```python
from build123d import *

# Parameters (mm, degrees)
SKETCH1_W           = 126
SKETCH1_H           = 126
BOSS_EXTRUDE1_DEPTH = 5
SKETCH3_R           = 12.5
BOSS_EXTRUDE2_DEPTH = 7.5
SKETCH4_R           = 2.95
CUT_EXTRUDE1_DEPTH  = 11.5
SKETCH6_R           = 2.5
CUT_EXTRUDE2_DEPTH  = 179.628805068
CHAMFER1_SIZE       = 10
CHAMFER1_SIZE_2     = 7.26542528
SKETCH8_W           = 13
SKETCH8_H           = 63.879672954
SKETCH8_H_2         = 19
CUT_EXTRUDE3_DEPTH  = 179.348675353
SKETCH9_R           = 30
CUT_EXTRUDE4_DEPTH  = 179.348675353
SKETCH11_W          = 2
SKETCH11_H          = 2
CUT_EXTRUDE5_DEPTH  = 3


with BuildPart() as part:
    # Sketch1 → Boss-Extrude1 (new body)
    with BuildSketch(Plane(origin=(0, 0, 0), x_dir=(1, 0, 0), z_dir=(0, 1, 0))):
        with Locations((63, 63)):
            Rectangle(SKETCH1_W, SKETCH1_H)
    extrude(amount=BOSS_EXTRUDE1_DEPTH)

    # Sketch3 → Boss-Extrude2 (add)
    with BuildSketch(Plane(origin=(0, 5, 0), x_dir=(1, 0, 0), z_dir=(0, 1, 0))):
        with Locations(Location((108.6, 108.6, 0), (0, 0, 90))):
            Circle(SKETCH3_R)
    extrude(amount=BOSS_EXTRUDE2_DEPTH)

    # Sketch4 → Cut-Extrude1 (cut)
    with BuildSketch(Plane.XZ):
        with Locations(Location((108.6, -108.6, 0), (0, 0, 270))):
            Circle(SKETCH4_R)
    extrude(amount=-CUT_EXTRUDE1_DEPTH, mode=Mode.SUBTRACT)

    # Sketch6 → Cut-Extrude2 (cut, through all)
    with BuildSketch(Plane(origin=(0, 12.5, 0), x_dir=(1, 0, 0), z_dir=(0, 1, 0))):
        with Locations(Location((108.6, 108.6, 0), (0, 0, 270))):
            Circle(SKETCH6_R)
    extrude(amount=-CUT_EXTRUDE2_DEPTH, mode=Mode.SUBTRACT)

    # Chamfer1
    # the kernel refuses this chamfer: 10, 7.26542528 mm, written as the material it takes off along each edge
    with BuildSketch(Plane(origin=(108.6, 12.5, -108.6), x_dir=(0, 0, -1), z_dir=(1, 0, 0))) as chamfer1_piece_1_section:
        Polygon((12.5, -CHAMFER1_SIZE), (12.5 - CHAMFER1_SIZE_2, 0), (12.5, 0), align=None)
    chamfer1_piece_1 = revolve(axis=Axis((108.6, 12.5, -108.6), (0, 1, 0)), mode=Mode.PRIVATE)
    chamfer1_piece_1 = split(chamfer1_piece_1, bisect_by=Plane(origin=(108.6, 5, -100.650989912), z_dir=(0, 1, 0)), keep=Keep.TOP, mode=Mode.PRIVATE)
    add(chamfer1_piece_1, mode=Mode.SUBTRACT)

    # Sketch8 → Cut-Extrude3 (cut, through all)
    with BuildSketch(Plane(origin=(0, 5, 0), x_dir=(1, 0, 0), z_dir=(0, 1, 0))):
        with Locations((107.763328316, 61.0093315)):
            Rectangle(SKETCH8_W, SKETCH8_H)
        with Locations((107.763328316, 14.5)):
            Rectangle(SKETCH8_W, SKETCH8_H_2)
    extrude(amount=-CUT_EXTRUDE3_DEPTH, mode=Mode.SUBTRACT)

    # Sketch9 → Cut-Extrude4 (cut, through all)
    with BuildSketch(Plane(origin=(0, 5, 0), x_dir=(1, 0, 0), z_dir=(0, 1, 0))):
        with Locations(Location((50.837155032, 48.974583989, 0), (0, 0, 270))):
            Circle(SKETCH9_R)
    extrude(amount=-CUT_EXTRUDE4_DEPTH, mode=Mode.SUBTRACT)

    # Sketch11 → Cut-Extrude5 (cut)
    with BuildSketch(Plane(origin=(0, 5, 0), x_dir=(1, 0, 0), z_dir=(0, 1, 0))):
        with Locations((50.837155032, 82.738467737)):
            Rectangle(SKETCH11_W, SKETCH11_H)
        with Locations((50.837155032, 15.21070024)):
            Rectangle(SKETCH11_W, SKETCH11_H)
    extrude(amount=-CUT_EXTRUDE5_DEPTH, mode=Mode.SUBTRACT)


solid = part.part
```
The listing builds one solid part. Answer for the finished solid, in the listing's coordinates (mm). A direction names the side the tool comes from. Coordinates: 2 decimals unless noted, no trailing zeros. Loops run counter-clockwise (first coordinate to the right, second up) from the corner with the lowest first, then second, coordinate; pieces in that order, holes last. Notation, with made-up numbers: (-2.5, -31.5) - (20.5, -31.5) arc R27 ccw to (20.5, -5.5) - close; hole circle Ø4 at (33.5, 32). An arc over 180 degrees is marked (long way). Use a Markdown table: item, result. Add a question column.
1) Find the intervals of material crossed by line 1 (X direction, y = 1.75, z = -17); line 2 (X direction, y = 2.25, z = -57); line 3 (Y direction, x = 86, z = -25), in increasing order.
2) The part is cut by section A-A, the plane z = -9. Give the vertices of the cut face in (x, y).
3) The mould has two halves that part along X. Classify faces 4 (the flat face through (62, 2, 0)), 5 (the conical face through (111.95, 12.14, -104.24)), 6 (the flat face through (108, 3, -92.949)), 7 (the flat face through (126, 2, -62)): released by +X, released by -X, zero draft, split by the parting line, or undercut.
4) The part is cut by section B-B, the plane x = 108.6. Give the vertices of the cut face in (y, z), and give its area (3 significant figures).
5) For faces 1 (the flat face through (108, 11.5, -106)), 2 (the flat face through (101.263, 3, -61)), 3 (the flat face through (111, 12.5, -110)), determine the directions among +Z, -Z, +X, -X, +Y, -Y from which every point of the face is accessible in a straight line to the end or side of a thin tool.
6) The part is cut by section C-C, the plane x = 54. Give the vertices of the cut face in (y, z), and give its area (3 significant figures).
7) The part is cut by section D-D, the plane z = -72.5. Give the vertices of the cut face in (x, y), and give its area (3 significant figures).
8) Given pin 1 (4 mm diameter, centred on y = 1.5, z = -15, fed in from -X); pin 2 (8 mm diameter, centred on x = 86, z = -106.5, fed in from +Y), each flat-ended and moving along its own axis, determine where each tip first touches the part or whether it passes through.
Here are the results:
| question | item | result |
|---|---|---|
| 1 | line 1 | x = 0 to 101.26, 114.26 to 126 |
| 1 | line 2 | x = 0 to 21.93, 79.74 to 101.26, 114.26 to 126 |
| 1 | line 3 | y = 0 to 5 |
| 2 | outline | (0, 0) - (101.26, 0) - (101.26, 5) - (0, 5) - close; (114.26, 0) - (126, 0) - (126, 5) - (114.26, 5) - close |
| 3 | face 4 | zero draft |
| 3 | face 5 | split by the parting line |
| 3 | face 6 | undercut |
| 3 | face 7 | released by +X |
| 4 | outline | (0, -126) - (5, -126) - (5, -119.28) - (12.5, -113.83) - (12.5, -111.1) - (11.5, -111.1) - (11.5, -111.55) - (0, -111.55) - close; (0, -105.65) - (11.5, -105.65) - (11.5, -106.1) - (12.5, -106.1) - (12.5, -103.37) - (5, -97.92) - (5, -92.95) - (0, -92.95) - close; (0, -29.07) - (5, -29.07) - (5, -24) - (0, -24) - close; (0, -5) - (5, -5) - (5, 0) - (0, 0) - close |
| 4 | area | 262 mm^2 |
| 5 | face 1 | -Y |
| 5 | face 2 | +Y, -Y |
| 5 | face 3 | +Z, -Z, +X, -X, +Y |
| 6 | outline | (0, -126) - (5, -126) - (5, -78.81) - (0, -78.81) - close; (0, -19.14) - (5, -19.14) - (5, 0) - (0, 0) - close |
| 6 | area | 332 mm^2 |
| 7 | outline | (0, 0) - (32.22, 0) - (32.22, 5) - (0, 5) - close; (69.45, 0) - (101.26, 0) - (101.26, 5) - (69.45, 5) - close; (114.26, 0) - (126, 0) - (126, 5) - (114.26, 5) - close |
| 7 | area | 379 mm^2 |
| 8 | pin 1 | stops at x = 0 |
| 8 | pin 2 | stops at y = 5 |
